```python
from build123d import *

# Parameters (mm, degrees)
SKETCH1_R                = 31.980898523
SKETCH1_R_2              = 25.45
BOSS_EXTRUDE1_DEPTH      = 20
SKETCH2_R                = 31.980898523
BOSS_EXTRUDE2_DEPTH      = 2
SKETCH3_R                = 5.114403944
BOSS_EXTRUDE3_DEPTH      = 1.5
BOSS_EXTRUDE3_DEPTH_BACK = 1.5


with BuildPart() as part:
    # Sketch1 → Boss-Extrude1 (new body)
    with BuildSketch(Plane.XY):
        Circle(SKETCH1_R)
        Circle(SKETCH1_R_2, mode=Mode.SUBTRACT)
    extrude(amount=BOSS_EXTRUDE1_DEPTH)

    # Sketch2 → Boss-Extrude2 (add)
    with BuildSketch(Plane.XY.offset(20)):
        Circle(SKETCH2_R)
    extrude(amount=BOSS_EXTRUDE2_DEPTH)

    # Sweep2: sweep along a path in Sketch4
    with BuildLine(Plane(origin=(0, 0, 0), x_dir=(0, 0, -1), z_dir=(1, 0, 0))) as sweep2_path:
        Line((-22, 0), (-56.496170036, 0))
        Line((-56.496170036, 0), (-56.496170036, -8.454631323))
    # Sketch3 → Sweep2 (sweep)
    with BuildSketch(Plane.XY.offset(22)):
        Circle(SKETCH3_R)
    sweep(path=sweep2_path.line, transition=Transition.RIGHT)

    # Sketch5 → Boss-Extrude3 (add, two sides)
    with BuildSketch(Plane(origin=(0, 0, 0), x_dir=(0, 0, -1), z_dir=(1, 0, 0))) as boss_extrude3_sk:
        with BuildLine():
            Line((-36.150092228, 0), (-36.150092228, 5.823788286))
            ThreePointArc((-36.150092228, 5.823788286), (-37.028771884, 7.94510863), (-39.150092228, 8.823788286))
            Line((-39.150092228, 8.823788286), (-40.746223013, 8.823788286))
            ThreePointArc((-40.746223013, 8.823788286), (-42.867543357, 9.702467943), (-43.746223013, 11.823788286))
            Line((-43.746223013, 11.823788286), (-43.746223013, 12.038804384))
            ThreePointArc((-43.746223013, 12.038804384), (-42.867543357, 14.160124727), (-40.746223013, 15.038804384))
            Line((-40.746223013, 15.038804384), (-34.162733631, 15.038804384))
            ThreePointArc((-34.162733631, 15.038804384), (-32.041413287, 14.160124727), (-31.162733631, 12.038804384))
            Line((-31.162733631, 12.038804384), (-31.162733631, 0))
            Line((-31.162733631, 0), (-36.150092228, 0))
        make_face()
    extrude(amount=BOSS_EXTRUDE3_DEPTH)
    extrude(boss_extrude3_sk.sketch, amount=-BOSS_EXTRUDE3_DEPTH_BACK)


solid = part.part
```
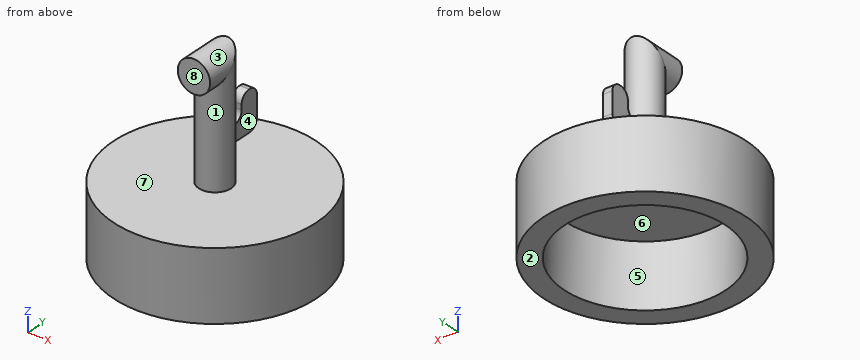
The listing builds one solid part. Answer for the finished solid, in the listing's coordinates (mm). Face numbers are marked on the shaded views. A direction names the side the tool comes from. Give positions to 0.01 mm unless a question says otherwise; leave off trailing zeros. Order: outer loops, then holes, each group sorted by start corner. A loop starts at its lowest first (then second) coordinate and runs counter-clockwise, first axis right, second up. Notation, with made-up numbers: M 33.5,73.5 L 78.5,73.5 A32 ccw 78.5,107.5 Z; hole C -11,77.25 d10. An arc over 180 degrees is marked long. Put each result on its own line as item: value. Start each with the question number.
Item 1: Find the intervals of material crossed by line 1 along Y through (x, z) = (0, 10); line 2 along Z through (x, y) = (-9.5, -13.5); line 3 along Z through (x, y) = (22.5, 14.5), in increasing order.
Item 2: The part is cut by section D-D, the plane z = 53. Determine the outline of the cut face in (x, y), and give its area (3 significant figures).
Item 3: Which of the six approach directions +Z, -Z, +X, -X, +Y, -Y give full straight-line access (tool end or side, diameter ignored) to the marked faces 1, 2, 3 and 4?
Item 4: The part is cut by section A-A, the plane x = 0. Determine the outline of the cut face in (y, z), and give its area (3 significant figures).
Item 5: Flat-ended cylindrical pins translate along their axes: P1, Ø6, axis at x = 24, z = 11.5, coming from the +Y side; P2, Ø1.8, axis at x = 0.5, z = 40.5, coming from the -Y side; P3, Ø0.9, axis at x = -0.5, y = 8.5, coming from the -Z side. Find the tip coordinate at first contact, or state that the pin passes through.
Item 6: The part is cut by section B-B, the plane z = 19. Determine the outline of the cut face in (x, y), and give its area (3 significant figures).
Item 7: The part is cut by section C-C, the plane y = 3. Determine the outline of the cut face in (x, z), and give its area (3 significant figures).
Item 8: For a pull along Y with two mould halves and no side action, classify the marked faces 5, 6, 7 and 8 as +Y half, -Y half, draft (parallel to the pull), parting line (faces both ways), or undercut.
Answer key:
1. line 1: y = -31.98 to -25.45, 25.45 to 31.98
1. line 2: z = 20 to 22
1. line 3: z = 0 to 22
2. outline: M -3.73,-8.45 L 3.73,-8.45 L 3.73,-3.5 A5.11 ccw long -3.73,-3.5 Z
2. area: 111 mm²
3. face 1: none
3. face 2: -Z, +X, -X, +Y, -Y
3. face 3: -Y
3. face 4: +Z, +X, +Y
4. outline: M -31.98,0 L -25.45,0 L -25.45,20 L 25.45,20 L 25.45,0 L 31.98,0 L 31.98,22 L 5.11,22 L 5.11,31.16 L 12.04,31.16 A3 ccw 15.04,34.16 L 15.04,40.75 A3 ccw 12.04,43.75 L 11.82,43.75 A3 ccw 8.82,40.75 L 8.82,39.15 A3 cw 5.82,36.15 L 5.11,36.15 L 5.11,61.61 L -8.45,61.61 L -8.45,51.38 L -5.11,51.38 L -5.11,22 L -31.98,22 Z
4. area: 921 mm²
5. P1: stops at y = 24.12
5. P2: stops at y = -5.11
5. P3: stops at z = 20
6. outline: C 0,0 d63.96; hole C 0,0 d50.9
6. area: 1,180 mm²
7. outline: M -31.84,0 L -25.27,0 L -25.27,20 L 25.27,20 L 25.27,0 L 31.84,0 L 31.84,22 L 4.14,22 L 4.14,59.5 A5.11 ccw -4.14,59.5 L -4.14,22 L -31.84,22 Z
7. area: 713 mm²
8. face 5: undercut
8. face 6: undercut
8. face 7: draft
8. face 8: -Y half
